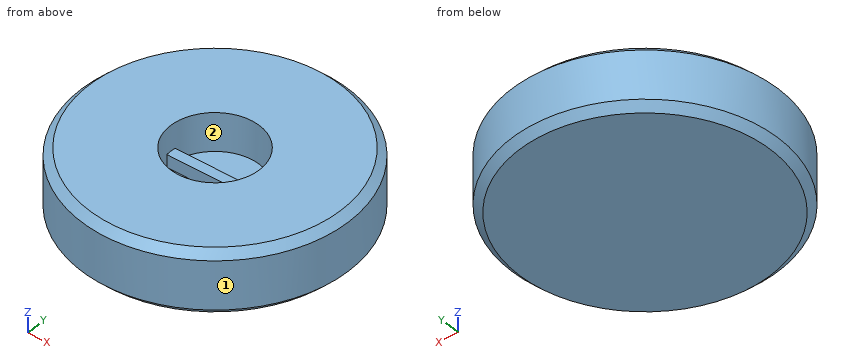
from build123d import *

# Parameters (mm, degrees)
F0_R     = 10.5
F1_DEPTH = 5
F2_R     = 3.5
F3_DEPTH = 3
F4_W     = 8
F4_H     = 0.8
F5_DEPTH = 1
F6_SIZE  = 0.6


with BuildPart() as f1:
    # F0 (on Top) → F1 (new body)
    with BuildSketch(Plane.XY):
        Circle(F0_R)
    extrude(amount=F1_DEPTH)

    # F2 (on face) → F3 (cut)
    with BuildSketch(Plane.XY.offset(5)):
        Circle(F2_R)
    extrude(amount=-F3_DEPTH, mode=Mode.SUBTRACT)

    # F4 (on face) → F5 (join)
    with BuildSketch(Plane.XY.offset(2)):
        Rectangle(F4_W, F4_H)
    extrude(amount=F5_DEPTH)

    # F6
    f6_edges = [f1.edges().sort_by_distance(p)[0] for p in [
        (-10.5, 0, 5),
        (-10.5, 0, 0),
    ]]
    chamfer(f6_edges, length=F6_SIZE)


solid = f1.part
Input: part model. Units: mm. Frame: model coordinates. Face numbers are marked on the shaded views. A direction names the side the tool comes from. Coordinates: 2 decimals unless noted, no trailing zeros. Loops run counter-clockwise (first coordinate to the right, second up) from the corner with the lowest first, then second, coordinate; pieces in that order, holes last.
(1) Section B-B on z = 2.65. Return the cut outline in (x, y), then the cut area to 3 significant figures.
(2) Section C-C on x = 0. Return the cut outline in (y, z).
(3) First-contact query: pin 1 Ø0.6 at (x, y) = (1, 0) entering from +Z; pin 2 Ø2 at (y, z) = (5.5, 3.5) entering from -X. Flat tips, straight axial feed; report the tip coordinate or a pass-through.
(4) Material intervals for probe 1 along Y at (x, z) = (0, 4.25); probe 2 along Y at (x, z) = (-0.5, 2.1); probe 3 along Z at (x, y) = (-0.75, -1.75), sorted ascending.
(5) Set-up query: the marked faces 1 and 2. Return all of +Z, -Z, +X, -X, +Y, -Y with unobstructed straight access to the full face (end or side cutting, diameter ignored); none if empty.
(6) Section A-A on y = 0. Return the cut outline in (x, z).
Data:
1. outline: circle Ø21 at (0, 0); hole (-3.48, -0.4) arc R3.5 ccw to (3.48, -0.4) - close; hole (-3.48, 0.4) - (3.48, 0.4) arc R3.5 ccw to start
1. area: 313 mm2
2. outline: (-10.5, 0.6) - (-9.9, 0) - (9.9, 0) - (10.5, 0.6) - (10.5, 4.4) - (9.9, 5) - (3.5, 5) - (3.5, 2) - (0.4, 2) - (0.4, 3) - (-0.4, 3) - (-0.4, 2) - (-3.5, 2) - (-3.5, 5) - (-9.9, 5) - (-10.5, 4.4) - close
3. pin 1: stops at z = 3
3. pin 2: stops at x = -9.49
4. probe 1: y = -10.5 to -3.5, 3.5 to 10.5
4. probe 2: y = -10.49 to -3.46, -0.4 to 0.4, 3.46 to 10.49
4. probe 3: z = 0 to 2
5. face 1: +Z, -Z
5. face 2: +Z
6. outline: (-10.5, 0.6) - (-9.9, 0) - (9.9, 0) - (10.5, 0.6) - (10.5, 4.4) - (9.9, 5) - (3.5, 5) - (3.5, 3) - (-3.5, 3) - (-3.5, 5) - (-9.9, 5) - (-10.5, 4.4) - close
